The listing builds one solid part. Answer for the finished solid, in the listing's coordinates (mm). A direction names the side the tool comes from. Give positions to 0.01 mm unless a question says otherwise; leave off trailing zeros. Order: outer loops, then holes, each group sorted by start corner. A loop starts at its lowest first (then second) coordinate and runs counter-clockwise, first axis right, second up. Notation, with made-up numbers: (8, 25.25) -> (17, 25.25) arc R36 ccw to (17, 63.25) -> close; hole circle Ø11 at (38, 40). An arc over 180 degrees is marked (long way). Write item = value, one per line. Start each with the question number.
```python
from build123d import *

# Parameters (mm, degrees)
BOSS_EXTRUDE1_DEPTH = 3
CUT_EXTRUDE1_DEPTH  = 3
SKETCH4_R           = 1.55
CUT_EXTRUDE4_DEPTH  = 3
SKETCH5_R           = 1.55
CUT_EXTRUDE6_DEPTH  = 3


with BuildPart() as part:
    # Sketch1 → Boss-Extrude1 (new body)
    with BuildSketch(Plane.XY):
        with BuildLine():
            Line((-58.058617241, 24.191090517), (5.941382759, 24.191090517))
            ThreePointArc((5.941382759, 24.191090517), (15.941382759, 14.191090517), (5.941382759, 4.191090517))
            Line((5.941382759, 4.191090517), (-58.058617241, 4.191090517))
            ThreePointArc((-58.058617241, 4.191090517), (-68.058617241, 14.191090517), (-58.058617241, 24.191090517))
        make_face()
    extrude(amount=BOSS_EXTRUDE1_DEPTH)

    # Sketch2 → Cut-Extrude1 (cut)
    with BuildSketch(Plane.XY.offset(3)):
        with BuildLine():
            Line((5.520256561, 17.941090517), (-10.129743439, 16.183590517))
            ThreePointArc((-10.129743439, 16.183590517), (-11.911009757, 14.191090517), (-10.129743439, 12.198590517))
            Line((-10.129743439, 12.198590517), (5.520256561, 10.441090517))
            ThreePointArc((5.520256561, 10.441090517), (9.714954976, 14.191090517), (5.520256561, 17.941090517))
        make_face()
    extrude(amount=-CUT_EXTRUDE1_DEPTH, mode=Mode.SUBTRACT)

    # Sketch4 → Cut-Extrude4 (cut)
    with BuildSketch(Plane(origin=(9.979459273, 1.433252018, 3), x_dir=(1, 0, 0), z_dir=(0, 0, 1))):
        with Locations((-40.038076514, 12.757838499)):
            Circle(SKETCH4_R)
    extrude(amount=-CUT_EXTRUDE4_DEPTH, mode=Mode.SUBTRACT)

    # Sketch5 → Cut-Extrude6 (cut)
    with BuildSketch(Plane(origin=(-9.979459273, 1.433252018, 0), x_dir=(-1, 0, 0), z_dir=(0, 0, -1))):
        with Locations((48.079157968, 12.757838499)):
            Circle(SKETCH5_R)
    extrude(amount=-CUT_EXTRUDE6_DEPTH, mode=Mode.SUBTRACT)


solid = part.part
```
Item 1: A cutting plane is placed at B-B, the plane y = 11.5. Write down the section's boundary in (x, z), plus the area to 3 significant figures.
Item 2: The mould has two halves that part along Y. Classify faces 1 (the flat face through (-2.41, 11.33, 1.52)), 2 (the flat face through (-27, 24.191, 1)), 3 (the flat face through (-25, 14, 0)): +Y half, -Y half, draft (parallel to the pull), parting line (faces both ways), or undercut.
Item 3: Consider L1, parallel to Y at x = -10, z = 1.25; L2, parallel to Y at x = 6, z = 2.35; L3, parallel to X at y = 18, z = 2.4. Determine where each line is inside the solid, lowest interval first. Write a range as from..to.
Item 4: Which of the six approach directions +Z, -Z, +X, -X, +Y, -Y give full straight-line access (tool end or side, diameter ignored) to faces 4 (the cylindrical face through (15.94, 14.41, 1.48)), 5 (the flat face through (-2.195, 17.075, 1.521))?
Item 5: A cutting plane is placed at D-D, the plane y = 20. Write down the section's boundary in (x, z).
Item 6: A cutting plane is placed at C-C, the plane z = 1.75. Write down the section's boundary in (x, y).
Item 7: A cutting plane is placed at A-A, the plane x = -4. Write down the section's boundary in (y, z), plus the area to 3 significant figures.
Check values:
q1.outline = (-67.69, 0) -> (-3.91, 0) -> (-3.91, 3) -> (-67.69, 3) -> close; (8.59, 0) -> (15.57, 0) -> (15.57, 3) -> (8.59, 3) -> close
q1.area = 212 mm^2
q2.face_1 = undercut
q2.face_2 = +Y half
q2.face_3 = draft
q3.L1 = 4.19..12.18, 16.2..24.19
q3.L2 = 4.19..10.42, 17.96..24.19
q3.L3 = -67.3..15.19
q4.face_4 = +Z, -Z, +X
q4.face_5 = +Z, -Z
q5.outline = (-66.2, 0) -> (14.08, 0) -> (14.08, 3) -> (-66.2, 3) -> close
q6.outline = (-58.06, 4.19) -> (5.94, 4.19) arc R10 ccw to (5.94, 24.19) -> (-58.06, 24.19) arc R10 ccw to start; hole circle Ø3.1 at (-58.06, 14.19); hole circle Ø3.1 at (-30.06, 14.19); hole (-10.13, 12.2) -> (5.52, 10.44) arc R3.77 ccw (long way) to (5.52, 17.94) -> (-10.13, 16.18) arc R2.01 ccw to start
q7.outline = (4.19, 0) -> (11.51, 0) -> (11.51, 3) -> (4.19, 3) -> close; (16.87, 0) -> (24.19, 0) -> (24.19, 3) -> (16.87, 3) -> close
q7.area = 43.9 mm^2
